Could you check a few things on this drawing? It's one solid part, dimensions in mm from its lowest x, y, z. Give positions to 0.01 mm unless a question says otherwise; leave off trailing zeros. Order: outer loops, then holes, each group sorted by start corner. A loop starts at its lowest first (then second) coordinate and runs counter-clockwise, first axis right, second up. Notation, with made-up numbers: M 55.5,66 L 86.5,66 A24 ccw 86.5,78 Z; hole C 78.25,-26 d4. An arc over 180 degrees is marked long. Use one line per item in the form item = value.
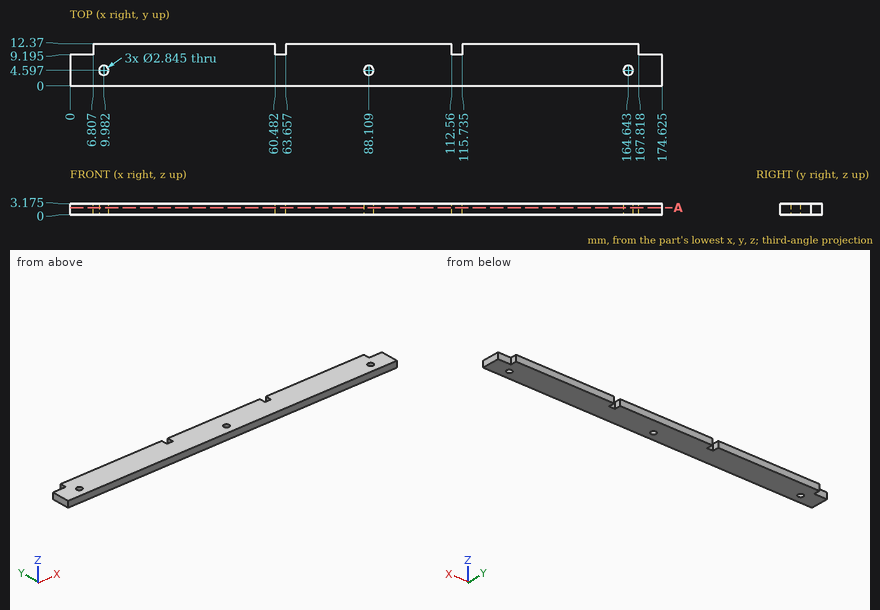
Q1. I need wall thicknesses on L1, parallel to X at y = 9.5, z = 1.9 (1 decimal); L2, parallel to X at y = 4.25, z = 1.5 (1 decimal); L3, parallel to Y at x = 63.5, z = 3.05 (1 decimal). Which ranges of each line are inside material? Lowest first, please.
Found:
L1 = 6.8 to 60.5, 63.7 to 112.6, 115.7 to 167.8
L2 = 0 to 8.6, 11.4 to 86.7, 89.5 to 163.3, 166 to 174.6
L3 = 0 to 9.2
Q2. I'm going to push flat-ended pins straight in: pin 1 Ø1 at (x, z) = (171.5, 2) entering from +Y (1 decimal); pin 2 Ø3.5 at (x, y) = (9.98, 4.6) entering from -Z; pin 3 Ø1.6 at (y, z) = (11.5, 1.5) entering from -X; pin 4 Ø1.6 at (y, z) = (11.5, 2.5) entering from +X. Where does each tip first touch, or does it pass through?
Found:
pin_1 = 9.2
pin_2 = 0
pin_3 = 6.81
pin_4 = 167.82
Q3. I want a section at A-A on z = 2.1. Write out the boundary of the cut face in (x, y) (1 decimal), then the cut area to 3 significant figures.
Found:
outline = M 0,0 L 174.6,0 L 174.6,9.2 L 167.8,9.2 L 167.8,12.4 L 115.7,12.4 L 115.7,9.2 L 112.6,9.2 L 112.6,12.4 L 63.7,12.4 L 63.7,9.2 L 60.5,9.2 L 60.5,12.4 L 6.8,12.4 L 6.8,9.2 L 0,9.2 Z; hole C 10,4.6 d2.8; hole C 88.1,4.6 d2.8; hole C 164.6,4.6 d2.8
area = 2,080 mm²
